Part model, mm, in its own coordinate system. Give positions to 0.01 mm unless a question says otherwise; leave off trailing zeros. Write each loop counter-clockwise with the first axis right and the second up, starting at its lowest first coordinate (ties: lowest second). Pieces come first, ordered by that corner, then holes. Notation, with made-up numbers: (80.5, 49) - (116.5, 49) arc R9 cw to (116.5, 58) - close; hole circle Ø7 at (38.5, 19.5). An arc over 180 degrees is marked (long way). Answer as a JSON object with one key per item and string values. Group by question number.
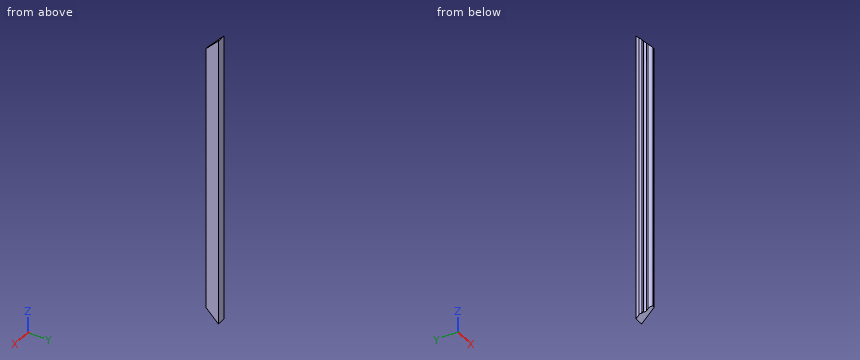
```python
from build123d import *

# Parameters (mm, degrees)
BASE_EXTRUDE_DEPTH = 315
CUT_EXTRUDE1_DEPTH = 328.294614629


with BuildPart() as part:
    # Sketch1 → Base-Extrude (new, symmetric)
    with BuildSketch(Plane.XY):
        with BuildLine():
            Line((17.889139296, 87.044491269), (-1.453845178, 87.044491269))
            Line((-1.453845178, 87.044491269), (-1.453845178, 80.35203196))
            ThreePointArc((-1.453845178, 80.35203196), (-0.32181751, 77.619075411), (2.411139039, 76.487047743))
            Line((2.411139039, 76.487047743), (2.411139039, 73.52781514))
            ThreePointArc((2.411139039, 73.52781514), (5.658603705, 72.483207804), (7.688030184, 69.741190405))
            Line((7.688030184, 69.741190405), (7.688030184, 66.961115937))
            ThreePointArc((7.688030184, 66.961115937), (9.575663464, 62.192626492), (14.215671126, 60.00814031))
            Line((14.215671126, 60.00814031), (17.889139296, 60.00814031))
            Line((17.889139296, 60.00814031), (17.889139296, 87.044491269))
        make_face()
    extrude(amount=BASE_EXTRUDE_DEPTH, both=True)

    # Sketch2 → Cut-Extrude1 (cut, symmetric)
    with BuildSketch(Plane(origin=(0, 0, 0), x_dir=(0, 0, -1), z_dir=(1, 0, 0))):
        Polygon((315, 87.044491269), (255, 27.044491269), (315, 27.044491269), align=None)
    cut_extrude1 = extrude(amount=CUT_EXTRUDE1_DEPTH, both=True, mode=Mode.SUBTRACT)

    # Mirror1: Cut-Extrude1 across plane
    add(cut_extrude1.mirror(Plane.XY), mode=Mode.SUBTRACT)


solid = part.part
```
1) Band-saw the part on A-A (z = -122). List the corners of the cut face in (x, y).
2) Probe line 1 (X direction, y = 67.25, z = -214.5); line 2 (Y direction, x = 2.25, z = 30); line 3 (Y direction, x = 13.75, z = 41.5). List the from-to ranges inside material, lowest first.
3) Drop flat-ended pins along their axis: P1, Ø2, axis at y = 68.5, z = -90.5, coming from the -X side; P2, Ø8, axis at x = 14, z = 182, coming from the -Y side; P3, Ø2.5, axis at y = 75, z = 2, coming from the -X side; P4, Ø3, axis at x = 5.5, z = -16.5, coming from the -Y side (3 decimals). Give the stop position or say it passes through.
Verdict:
{
 "1": {"outline": "(-1.45, 80.35) arc R3.86 ccw to (2.41, 76.49) - (2.41, 73.53) arc R5.57 cw to (7.69, 69.74) - (7.69, 66.96) arc R6.97 ccw to (14.22, 60.01) - (17.89, 60.01) - (17.89, 87.04) - (-1.45, 87.04) - close"},
 "2": {"line 1": "7.69 to 17.89", "line 2": "76.49 to 87.04", "line 3": "60.05 to 87.04"},
 "3": {"P1": "x = 7.69", "P2": "y = 60.01", "P3": "x = 2.41", "P4": "y = 71.115"}
}
